Input: part model. Units: mm. Frame: model coordinates. Round coordinates to 2 decimals unless told otherwise and drop trailing zeros. Loops run counter-clockwise (first coordinate to the right, second up) from the corner with the lowest first, then second, coordinate; pieces in that order, holes last. Notation, with made-up numbers: (6, -37) -> (24, -37) arc R19 ccw to (24, -30) -> close; hole circle Ø6 at (12, -20). An arc over 180 degrees is marked (long way). Answer as a JSON object with one key per item and string values.
Autodesk Inventor part; units mm, degrees
ref_plane "YZ Plane" through (0, 0, 0) normal (1, 0, 0) x (0, 1, 0)
ref_plane "XZ Plane" through (0, 0, 0) normal (0, 1, 0) x (-1, 0, 0)
ref_plane "XY Plane" through (0, 0, 0) normal (0, 0, 1) x (1, 0, 0)
sketch "Sketch1" plane through (0, 0, 0) normal (1, 0, 0) x (0, 1, 0)
  circle A0 centre (0, 0) radius 40
  dimension "d0" = 80
extrude "Extrusion1" add sketch "Sketch1" along normal blind 5
sketch "Sketch2" plane through (5, 0, 0) normal (1, 0, 0) x (0, 0, -1)
  circle A0 centre (30, 0) radius 3.5
  circle A1 centre (0, 0) radius 3.5
  circle A2 centre (0, 30) radius 3.5
  circle A3 centre (-30, 0) radius 3.5
  circle A4 centre (0, -30) radius 3.5
  circle A5 centre (-15, 25.9808) radius 3.5
  circle A6 centre (-15, -25.9808) radius 3.5
  dimension "d3" = 7
  dimension "d4" = 30
  dimension "d5" = 7
  dimension "d8" = 360
  dimension "d12" = 360
extrude "Extrusion2" cut sketch "Sketch2" against normal through all
properties part number "end effector Plate"
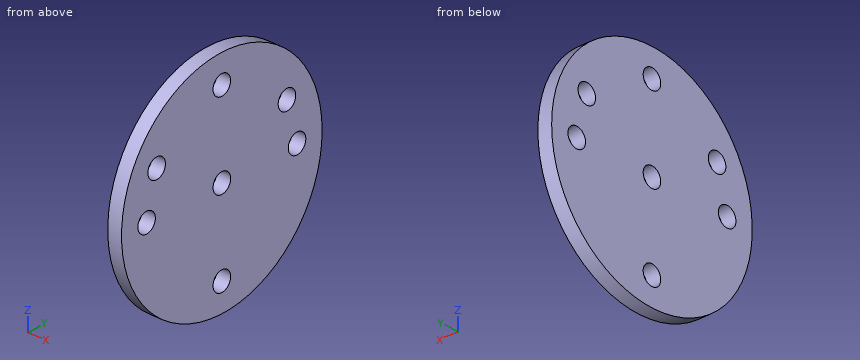
1) Contact query for a flat-ended pin moving along its axis: P1, Ø1, axis at x = 1.5, y = 15, coming from the +Z side. Output: stop coordinate, or through.
Output:
{"P1": "stops at z = 37.28"}
2) Section C-C, the plane z = 15. Output: boundary loops of the cut face in (x, y).
Output:
{"outline": "(0, -37.08) -> (5, -37.08) -> (5, -29.48) -> (0, -29.48) -> close; (0, -22.48) -> (5, -22.48) -> (5, 22.48) -> (0, 22.48) -> close; (0, 29.48) -> (5, 29.48) -> (5, 37.08) -> (0, 37.08) -> close"}
3) Section D-D, the plane y = -24. Output: boundary loops of the cut face in (x, z).
Output:
{"outline": "(0, -32) -> (5, -32) -> (5, 12.11) -> (0, 12.11) -> close; (0, 17.89) -> (5, 17.89) -> (5, 32) -> (0, 32) -> close"}
4) Ray query, probe 1 along Y at (x, z) = (1.5, -1); probe 2 along Z at (x, y) = (0.3, 3); probe 3 along Z at (x, y) = (0.55, -2). Return the intervals inside material, ascending.
Output:
{"probe 1": "y = -39.99 to -33.35, -26.65 to -3.35, 3.35 to 26.65, 33.35 to 39.99", "probe 2": "z = -39.89 to -31.8, -28.2 to -1.8, 1.8 to 28.2, 31.8 to 39.89", "probe 3": "z = -39.95 to -32.87, -27.13 to -2.87, 2.87 to 27.13, 32.87 to 39.95"}
5) Section A-A, the plane z = 0. Output: boundary loops of the cut face in (x, y), plus the area to 3 significant figures.
Output:
{"outline": "(0, -40) -> (5, -40) -> (5, -33.5) -> (0, -33.5) -> close; (0, -26.5) -> (5, -26.5) -> (5, -3.5) -> (0, -3.5) -> close; (0, 3.5) -> (5, 3.5) -> (5, 26.5) -> (0, 26.5) -> close; (0, 33.5) -> (5, 33.5) -> (5, 40) -> (0, 40) -> close", "area": "295 mm^2"}
